Print and shaded views of the part. All mm, measured from the part's lowest x, y and z. Coordinates: 2 decimals unless noted, no trailing zeros. Write each loop counter-clockwise with the first axis right and the second up, starting at its lowest first coordinate (ties: lowest second). Pieces come first, ordered by that corner, then holes. Notation, with made-up numbers: (-16.5, 44.25) -> (26.5, 44.25) arc R8 ccw to (26.5, 56.25) -> close; hole circle Ø7 at (32, 23.5). An arc over 180 degrees is marked (long way). Write item = value, one per line.
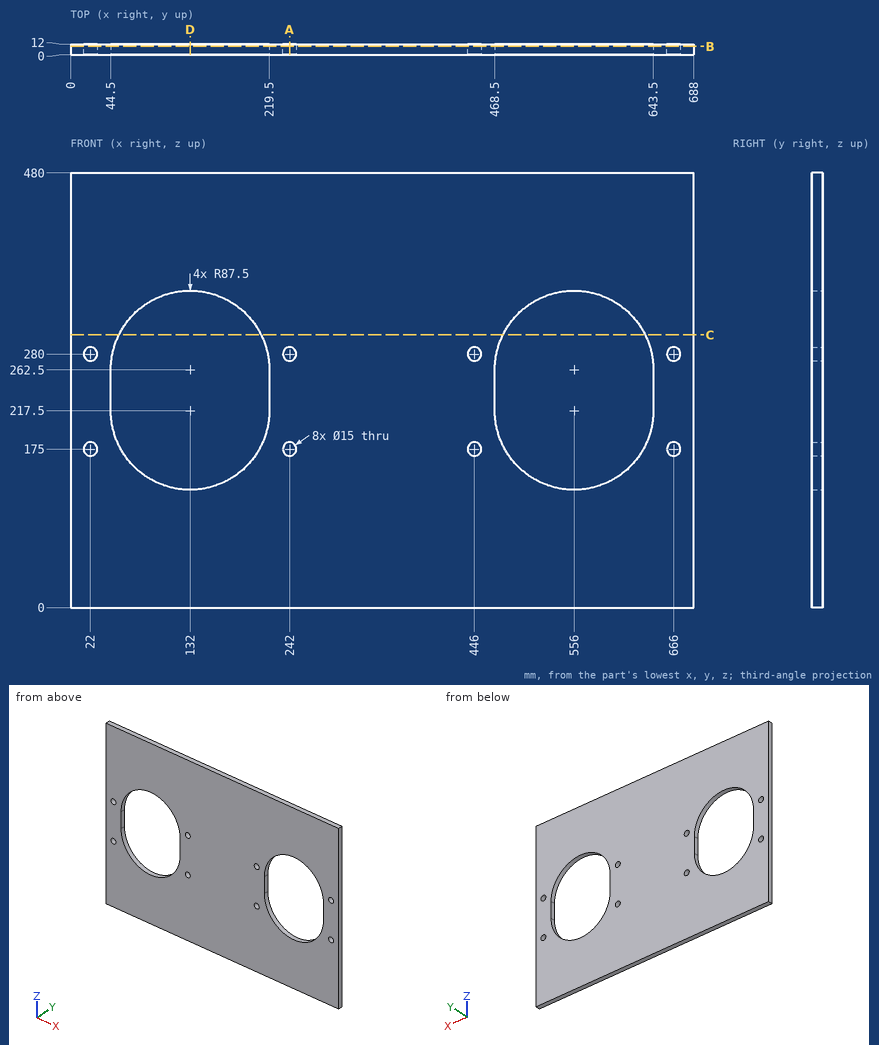
Q1. Saw through at B-B on y = 9.5. Count the separate pieces of the cut face and the enclosed holes in it, and give its area (3 significant figures).
Model answer:
separate_pieces = 1
enclosed_holes = 10
area = 265,000 mm²
Q2. Saw through at D-D on x = 132. Give the cut face in (y, z).
Model answer:
outline = (0, 0) -> (12, 0) -> (12, 130) -> (0, 130) -> close; (0, 350) -> (12, 350) -> (12, 480) -> (0, 480) -> close
Q3. Probe line 1 (Z direction, x = 22, y = 3.25); line 2 (X direction, y = 10.25, z = 232.5); line 3 (X direction, y = 5, z = 202). List the from-to ranges inside material, lowest first. Write a range as from..to.
Model answer:
line_1 = 0..167.5, 182.5..272.5, 287.5..480
line_2 = 0..44.5, 219.5..468.5, 643.5..688
line_3 = 0..45.88, 218.12..469.88, 642.12..688
Q4. Saw through at C-C on z = 301. Give the cut face in (x, y), and give its area (3 significant figures).
Model answer:
outline = (0, 0) -> (53.43, 0) -> (53.43, 12) -> (0, 12) -> close; (210.57, 0) -> (477.43, 0) -> (477.43, 12) -> (210.57, 12) -> close; (634.57, 0) -> (688, 0) -> (688, 12) -> (634.57, 12) -> close
area = 4,480 mm²
Q5. Pin check, flat tip, straight feed: pin 1 (12 mm diameter, centred on x = 666, z = 175, fed in from +Y). Stop position of the tip, or through.
Model answer:
pin_1 = through
Q6. Saw through at A-A on x = 242. Give the cut face in (y, z).
Model answer:
outline = (0, 0) -> (12, 0) -> (12, 167.5) -> (0, 167.5) -> close; (0, 182.5) -> (12, 182.5) -> (12, 272.5) -> (0, 272.5) -> close; (0, 287.5) -> (12, 287.5) -> (12, 480) -> (0, 480) -> close
